from build123d import *

# Parameters (mm, degrees)
F1_DEPTH = 80
F2_R     = 16
F3_DEPTH = 50.001
F4_R     = 9.5
F5_DEPTH = 119.001


with BuildPart() as f1:
    # F0 (on Front) → F1 (new body)
    with BuildSketch(Plane.XZ):
        Polygon((-29.880095, 26.308924), (-20.880095, 26.308924), (-20.880095, 136.308924), (11.119905, 136.308924), (11.119905, 26.308924), (20.119905, 26.308924), (20.119905, 145.308924), (-29.880095, 145.308924), align=None)
    extrude(amount=F1_DEPTH)

    # F2 (on face) → F3 (cut, through all)
    with BuildSketch(Plane(origin=(-29.880095, 0, 0), x_dir=(0, -1, 0), z_dir=(-1, 0, 0))):
        with Locations((40, 66.308924)):
            Circle(F2_R)
    extrude(amount=-F3_DEPTH, mode=Mode.SUBTRACT)

    # F4 (on face) → F5 (cut, through all)
    with BuildSketch(Plane.XY.offset(145.308924)):
        with Locations((-4.880095, -40)):
            Circle(F4_R)
    extrude(amount=-F5_DEPTH, mode=Mode.SUBTRACT)


solid = f1.part
The model under review builds one solid part; all positions refer to its coordinate system, in mm. A direction names the side the tool comes from. Round coordinates to 2 decimals unless told otherwise and drop trailing zeros. Order: outer loops, then holes, each group sorted by start corner. A loop starts at its lowest first (then second) coordinate and runs counter-clockwise, first axis right, second up. Notation, with made-up numbers: (50.5, 8.5) - (82.5, 8.5) arc R24 ccw to (82.5, 18.5) - close; hole circle Ø9 at (2, 29.5). An arc over 180 degrees is marked (long way). Use one line per item in the form item = value.
Q1. To check wall thickness, follow line 1 (Z direction, x = -26, y = -40); line 2 (X direction, y = -36, z = 116.5); line 3 (Z direction, x = -16, y = -75.5). State the ranges of each line that lie inside material, in increasing order.
Response values:
line_1 = 26.31 to 50.31, 82.31 to 145.31
line_2 = -29.88 to -20.88, 11.12 to 20.12
line_3 = 136.31 to 145.31
Q2. Clearance check with a flat-ended pin moving along its axis: P1, Ø4, axis at x = -8, y = -13, coming from the -Z side. State where the tip first meets the part, or that it passes through.
Response values:
P1 = 136.31
Q3. Add section C-C on z = 39. Give the boundary of the cut face in (x, y).
Response values:
outline = (-29.88, -80) - (-20.88, -80) - (-20.88, 0) - (-29.88, 0) - close; (11.12, -80) - (20.12, -80) - (20.12, 0) - (11.12, 0) - close
Q4. Tool access review of faces 4 (the flat face through (-25, -39, 26.309)), 5 (the flat face through (-20.88, -31, 81)): name each direction out of +Z, -Z, +X, -X, +Y, -Y from which nothing blocks a thin tool from reaching the whole face with its end or side.
Response values:
face_4 = -Z, +X, -X, +Y, -Y
face_5 = -Z, +Y, -Y
Q5. Add section D-D on z = 60. Give the boundary of the cut face in (x, y), then the cut area to 3 significant figures.
Response values:
outline = (-29.88, -80) - (-20.88, -80) - (-20.88, -54.7) - (-29.88, -54.7) - close; (-29.88, -25.3) - (-20.88, -25.3) - (-20.88, 0) - (-29.88, 0) - close; (11.12, -80) - (20.12, -80) - (20.12, -54.7) - (11.12, -54.7) - close; (11.12, -25.3) - (20.12, -25.3) - (20.12, 0) - (11.12, 0) - close
area = 911 mm^2
Q6. Mouldability with a two-part tool opening along X and no side actions: class faces 1 (the flat face through (20.12, -39, 85)), 2 (the cylindrical face through (15.557, -24.015, 67.012)), 3 (the flat face through (-9, -31, 136.309)) as pulls with the +X half, pulls with the -X half, needs draft (parallel to the pull), parting line crosses it, or undercut.
Response values:
face_1 = pulls with the +X half
face_2 = needs draft
face_3 = undercut
Q7. Add section B-B on x = -2. Give the boundary of the cut face in (y, z), then the cut area to 3 significant figures.
Response values:
outline = (-80, 136.31) - (-49.05, 136.31) - (-49.05, 145.31) - (-80, 145.31) - close; (-30.95, 136.31) - (0, 136.31) - (0, 145.31) - (-30.95, 145.31) - close
area = 557 mm^2
Q8. Add section A-A on y = -40. Give the boundary of the cut face in (x, z).
Response values:
outline = (-29.88, 26.31) - (-20.88, 26.31) - (-20.88, 50.31) - (-29.88, 50.31) - close; (-29.88, 82.31) - (-20.88, 82.31) - (-20.88, 136.31) - (-14.38, 136.31) - (-14.38, 145.31) - (-29.88, 145.31) - close; (4.62, 136.31) - (11.12, 136.31) - (11.12, 82.31) - (20.12, 82.31) - (20.12, 145.31) - (4.62, 145.31) - close; (11.12, 26.31) - (20.12, 26.31) - (20.12, 50.31) - (11.12, 50.31) - close
